CAD build for the part. Positions are in the model's coordinates, mm. Face numbers are marked on the shaded views. A direction names the side the tool comes from. Give positions to 0.01 mm unless a question says otherwise; leave off trailing zeros. Order: outer loops, then holes, each group sorted by start corner. A loop starts at its lowest first (then second) coordinate and runs counter-clockwise, first axis right, second up.
from build123d import *

# Parameters (mm, degrees)
SKETCH_1_R             = 12.5
EXTRUDE_1_DEPTH        = 15
SKETCH_1_3_R           = 12.5
CUT_EXTRUDE_1_DEPTH    = 8
FILLET_1_R             = 2
SHELL_1_T              = -1.5
CUT_EXTRUDE_2_DEPTH    = 8
PATTERN_START          = -1.5
PATTERN_LINEAR_6_DEPTH = 1.5


# Read off the part's stored shape, not the designer's step: 阵列(线性)6
with BuildPart() as part:
    # 草图1 → 凸台-拉伸1 (new body)
    # profile 1 of 2: a face of its own
    with BuildSketch(Plane(origin=(0, 0, 0), x_dir=(1, 0, 0), z_dir=(0, 1, 0))):
        with BuildLine():
            ThreePointArc((6.109515315, -38.6086173), (0, -23), (-6.109515315, -38.6086173))
            ThreePointArc((-6.109515315, -38.6086173), (-4.451858441, -45.825779601), (-10.568323275, -50))
            Line((-10.568323275, -50), (-26, -50))
            ThreePointArc((-26, -50), (-32.346826722, -46.870091432), (-33.72740661, -39.929447639))
            Line((-33.72740661, -39.929447639), (-28.151949957, -19.121560132))
            ThreePointArc((-28.151949957, -19.121560132), (-27.721159204, -13.070589863), (-29.573912969, -7.294161438))
            ThreePointArc((-29.573912969, -7.294161438), (-32.875929141, 1.074218994), (-34, 10))
            Line((-34, 10), (-34, 52))
            ThreePointArc((-34, 52), (-31.656854249, 57.656854249), (-26, 60))
            Line((-26, 60), (26, 60))
            ThreePointArc((26, 60), (31.656854249, 57.656854249), (34, 52))
            Line((34, 52), (34, 10))
            ThreePointArc((34, 10), (32.875929141, 1.074218994), (29.573912969, -7.294161438))
            ThreePointArc((29.573912969, -7.294161438), (27.721159204, -13.070589863), (28.151949957, -19.121560132))
            Line((28.151949957, -19.121560132), (33.72740661, -39.929447639))
            ThreePointArc((33.72740661, -39.929447639), (32.346826722, -46.870091432), (26, -50))
            Line((26, -50), (10.568323275, -50))
            ThreePointArc((10.568323275, -50), (4.451858441, -45.825779601), (6.109515315, -38.6086173))
        make_face()
        Circle(SKETCH_1_R, mode=Mode.SUBTRACT)
    # profile 2 of 2: a face of its own
    with BuildSketch(Plane(origin=(0, 0, 0), x_dir=(1, 0, 0), z_dir=(0, 1, 0))):
        Circle(SKETCH_1_R)
    extrude(amount=-EXTRUDE_1_DEPTH)

    # 草图1<3> → 切除-拉伸1 (cut)
    with BuildSketch(Plane(origin=(0, 0, 0), x_dir=(1, 0, 0), z_dir=(0, 1, 0))):
        with Locations(Location((0, 0, 0), (0, 0, 270))):
            Circle(SKETCH_1_3_R)
    extrude(amount=-CUT_EXTRUDE_1_DEPTH, mode=Mode.SUBTRACT)

    # 圆角1
    fillet_1_edges = [part.edges().sort_by_distance(p)[0] for p in [
        (0, -8, -12.5),
    ]]
    fillet(fillet_1_edges, radius=FILLET_1_R)

    # 抽壳1
    shell_1_openings = [part.faces().sort_by_distance(p)[0] for p in [
        (0, -15, -8.148675604),
    ]]
    offset(amount=SHELL_1_T, openings=shell_1_openings, kind=Kind.INTERSECTION)

    # 草图2 → 切除-拉伸2 (cut)
    with BuildSketch(Plane(origin=(0, 0, 0), x_dir=(1, 0, 0), z_dir=(0, 1, 0))):
        with BuildLine():
            Line((-28, 22.074023338), (-28, 50))
            ThreePointArc((-28, 50), (-26, 52), (-24, 50))
            Line((-24, 50), (-24, 22.074023338))
            ThreePointArc((-24, 22.074023338), (-26, 20.074023338), (-28, 22.074023338))
        make_face()
    extrude(amount=-CUT_EXTRUDE_2_DEPTH, mode=Mode.SUBTRACT)

    # 阵列(线性)6 outline → 阵列(线性)6 (cut)
    with BuildSketch(Plane(origin=(0, 0, 0), x_dir=(1, 0, 0), z_dir=(0, 1, 0)).offset(PATTERN_START)):
        with BuildLine():
            Line((24, 50), (24, 22.074023338))
            ThreePointArc((24, 22.074023338), (26, 20.074023338), (28, 22.074023338))
            Line((28, 22.074023338), (28, 50))
            ThreePointArc((28, 50), (26, 52), (24, 50))
        make_face()
        with BuildLine():
            Line((11, 50), (11, 26.574738582))
            ThreePointArc((11, 26.574738582), (13, 24.574738582), (15, 26.574738582))
            Line((15, 26.574738582), (15, 50))
            ThreePointArc((15, 50), (13, 52), (11, 50))
        make_face()
        with BuildLine():
            Line((-2, 50), (-2, 28))
            ThreePointArc((-2, 28), (0, 26), (2, 28))
            Line((2, 28), (2, 50))
            ThreePointArc((2, 50), (0, 52), (-2, 50))
        make_face()
        with BuildLine():
            Line((-15, 50), (-15, 26.574738582))
            ThreePointArc((-15, 26.574738582), (-13, 24.574738582), (-11, 26.574738582))
            Line((-11, 26.574738582), (-11, 50))
            ThreePointArc((-11, 50), (-13, 52), (-15, 50))
        make_face()
    extrude(amount=PATTERN_LINEAR_6_DEPTH, mode=Mode.SUBTRACT)


solid = part.part
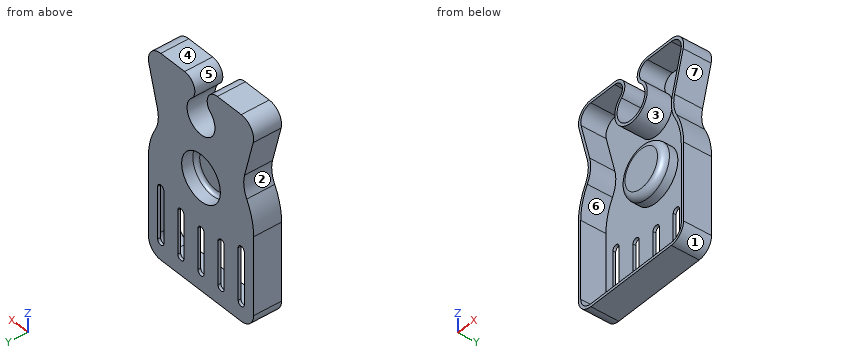
1. 3-axis set-ups, long thin cutter, end or side, ignore diameter. For the marked faces 5, 6 and 7: which of +Z, -Z, +X, -X, +Y, -Y reach the whole face in a straight line?
2. Pin check, flat tips, straight feed: P1, Ø6, axis at x = 7, z = 14.5, coming from the -Y side; P2, Ø10.5, axis at x = 3.5, z = 3.5, coming from the -Y side; P3, Ø6.5, axis at x = 3, z = -4, coming from the +Y side. Stop position of each tip, or through.
3. Mould opens along X. For the marked faces 1, 2, 3 and 4 say: released by +X, released by -X, zero draft, split by the parting line, or undercut.
4. Saw through at B-B on x = 0. Give the cut face in (y, z).
5. Wall check: line 1 (Z direction, x = 13, y = -9.25); line 2 (X direction, y = -4, z = -51); line 3 (X direction, y = -8.5, z = 32). Give the ranges that are in metal, low to high.
6. Saw through at C-C on x = 19.5. Give the cut face in (y, z), plus the area to 4 significant figures.
7. Saw through at D-D on y = -4.5. State how many separate pieces and enclosed holes the cut face has, plus the area to 3 significant figures.
8. Saw through at A-A on z = -42.5. Give the cut face in (x, y).
Reported:
1. face 5: +Y, -Y
1. face 6: -Y
1. face 7: +X, +Y, -Y
2. P1: stops at y = -8.34
2. P2: stops at y = -9.5
2. P3: stops at y = -8
3. face 1: released by +X
3. face 2: released by -X
3. face 3: undercut
3. face 4: zero draft
4. outline: (-15, -60) - (0, -60) - (0, -52) - (-1.5, -52) - (-1.5, -58.5) - (-15, -58.5) - close; (-15, 21.5) - (-1.5, 21.5) - (-1.5, 14) - (-6, 14) arc R3.5 ccw to (-9.5, 10.5) - (-9.5, -10.5) arc R3.5 ccw to (-6, -14) - (-1.5, -14) - (-1.5, -26) - (0, -26) - (0, -12.5) - (-6, -12.5) arc R2 cw to (-8, -10.5) - (-8, 10.5) arc R2 cw to (-6, 12.5) - (0, 12.5) - (0, 23) - (-15, 23) - close
5. line 1: z = -60 to -58.5, 48.5 to 50
5. line 2: x = -34 to -32.5, 32.5 to 34
5. line 3: x = -31.6 to -30.05, -10.5 to -9, 9 to 10.5, 30.05 to 31.6
6. outline: (-15, -60) - (0, -60) - (0, 50) - (-15, 50) - (-15, 48.5) - (-1.5, 48.5) - (-1.5, -58.5) - (-15, -58.5) - close
6. area: 205.5 mm2
7. separate pieces: 2
7. enclosed holes: 2
7. area: 717 mm2
8. outline: (-34, -15) - (-32.5, -15) - (-32.5, -1.5) - (-28, -1.5) - (-28, 0) - (-34, 0) - close; (-24, -1.5) - (-15, -1.5) - (-15, 0) - (-24, 0) - close; (-11, -1.5) - (-2, -1.5) - (-2, 0) - (-11, 0) - close; (2, -1.5) - (11, -1.5) - (11, 0) - (2, 0) - close; (15, -1.5) - (24, -1.5) - (24, 0) - (15, 0) - close; (28, -1.5) - (32.5, -1.5) - (32.5, -15) - (34, -15) - (34, 0) - (28, 0) - close
